Read the model definition and answer for the solid it produces. Units are mm, in the model's axes. Round coordinates to 2 decimals unless told otherwise and drop trailing zeros.
from build123d import *

# Parameters (mm, degrees)
SKETCH_1_R      = 4.25
EXTRUDE_1_DEPTH = 10
FILLET_1_R      = 30
FILLET_2_R      = 3


with BuildPart() as part:
    # 草图1 → 凸台-拉伸1 (new body)
    with BuildSketch(Plane(origin=(0, 0, 0), x_dir=(1, 0, 0), z_dir=(0, 1, 0))):
        Polygon((60, 0), (60, -55), (70, -55), (70, -70), (55, -70), (55, -60), (0, -60), (0, -300), (600, -300), (600, 0), align=None)
        with Locations(Location((103.5, -11, 0), (0, 0, 270))):
            Circle(SKETCH_1_R, mode=Mode.SUBTRACT)
        with Locations(Location((87.5, -11, 0), (0, 0, 270))):
            Circle(SKETCH_1_R, mode=Mode.SUBTRACT)
        with Locations(Location((103.5, -41, 0), (0, 0, 270))):
            Circle(SKETCH_1_R, mode=Mode.SUBTRACT)
        with Locations(Location((87.5, -41, 0), (0, 0, 270))):
            Circle(SKETCH_1_R, mode=Mode.SUBTRACT)
        with Locations(Location((16, -87.5, 0), (0, 0, 270))):
            Circle(SKETCH_1_R, mode=Mode.SUBTRACT)
        with Locations(Location((46, -87.5, 0), (0, 0, 270))):
            Circle(SKETCH_1_R, mode=Mode.SUBTRACT)
        with Locations(Location((16, -103.5, 0), (0, 0, 270))):
            Circle(SKETCH_1_R, mode=Mode.SUBTRACT)
        with Locations(Location((46, -103.5, 0), (0, 0, 270))):
            Circle(SKETCH_1_R, mode=Mode.SUBTRACT)
    extrude(amount=EXTRUDE_1_DEPTH)

    # 圆角1
    fillet_1_edges = [part.edges().sort_by_distance(p)[0] for p in [
        (600, 5, 300),
        (0, 5, 300),
        (600, 5, 0),
    ]]
    fillet(fillet_1_edges, radius=FILLET_1_R)

    # 圆角2
    fillet_2_edges = [part.edges().sort_by_distance(p)[0] for p in [
        (0, 5, 60),
        (55, 5, 60),
        (55, 5, 70),
        (70, 5, 70),
        (70, 5, 55),
        (60, 5, 55),
        (60, 5, 0),
    ]]
    fillet(fillet_2_edges, radius=FILLET_2_R)


solid = part.part
Q1. A flat-ended cylindrical pin translates along its axis: pin 1 (11 mm diameter, centred on x = 103.5, z = 41, fed in from +Y). Find the tip coordinate at first contact, or state that the pin passes through.
Outcome:
pin 1: stops at y = 10
Q2. Straight lines are drawn through the part: probe 1 along X at (y, z) = (8, 41); probe 2 along X at (y, z) = (3.25, 87.5); probe 3 along Z at (x, y) = (36, 9.75). For each, find the intervals that lie inside material, in ascending order.
Outcome:
probe 1: x = 60 to 83.25, 91.75 to 99.25, 107.75 to 600
probe 2: x = 0 to 11.75, 20.25 to 41.75, 50.25 to 600
probe 3: z = 60 to 300
Q3. A cutting plane is placed at A-A, the plane y = 2.5. Give the number of separate pieces and of enclosed holes in the cut face, plus the area to 3 significant figures.
Outcome:
separate pieces: 1
enclosed holes: 8
area: 175,000 mm2
